Verification items for the finished model (mm, model axes). Round coordinates to 2 decimals unless told otherwise and drop trailing zeros. Write each loop counter-clockwise with the first axis right and the second up, starting at its lowest first coordinate (ties: lowest second). Pieces come first, ordered by that corner, then holes. Notation, with made-up numbers: M 78.25,-4 L 98.25,-4 A15 ccw 98.25,22 Z; hole C 73.5,40 d6. An arc over 180 degrees is marked long. Use a Markdown table: item, result. Add a question column.
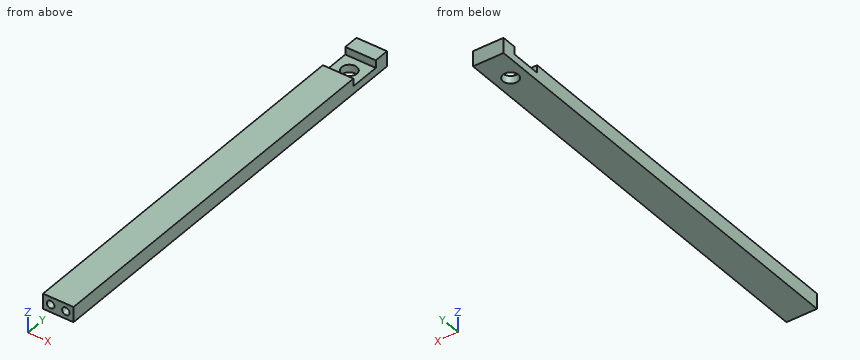
from build123d import *

# Parameters (mm, degrees)
SKETCH1_W           = 25.4
SKETCH1_H           = 12.7
BOSS_EXTRUDE1_DEPTH = 355.6
SKETCH2_W           = 6.35
SKETCH2_H           = 25.4
CUT_EXTRUDE1_DEPTH  = 357.732126392
SKETCH3_R           = 6.35
CUT_EXTRUDE2_DEPTH  = 357.562536591
SKETCH4_R           = 3.175
CUT_EXTRUDE3_DEPTH  = 25.4


with BuildPart() as part:
    # Sketch1 → Boss-Extrude1 (new body)
    with BuildSketch(Plane(origin=(0, 0, 0), x_dir=(1, 0, 0), z_dir=(0, 1, 0))):
        with Locations((12.7, 6.35)):
            Rectangle(SKETCH1_W, SKETCH1_H)
    extrude(amount=BOSS_EXTRUDE1_DEPTH)

    # Sketch2 → Cut-Extrude1 (cut, through all)
    with BuildSketch(Plane(origin=(25.4, 0, 0), x_dir=(0, 0, -1), z_dir=(1, 0, 0))):
        with Locations((3.175, 330.2)):
            Rectangle(SKETCH2_W, SKETCH2_H)
    extrude(amount=-CUT_EXTRUDE1_DEPTH, mode=Mode.SUBTRACT)

    # Sketch3 → Cut-Extrude2 (cut, through all)
    with BuildSketch(Plane.XY.offset(-6.35)):
        with Locations((12.7, 330.2)):
            Circle(SKETCH3_R)
    extrude(amount=-CUT_EXTRUDE2_DEPTH, mode=Mode.SUBTRACT)

    # Sketch4 → Cut-Extrude3 (cut)
    with BuildSketch(Plane.XZ):
        with Locations(Location((6.35, -6.35, 0), (0, 0, 270))):
            Circle(SKETCH4_R)
        with Locations(Location((19.05, -6.35, 0), (0, 0, 270))):
            Circle(SKETCH4_R)
    extrude(amount=-CUT_EXTRUDE3_DEPTH, mode=Mode.SUBTRACT)


solid = part.part
1. Cross-section at A-A on x = 12.7. Enter the section's corners in (y, z).
2. Scan lines: line 1 along X through (y, z) = (18.5, -6.35) (3 decimals); line 2 along X through (y, z) = (330.2, -9); line 3 along Y through (x, z) = (24.75, -3.5). Record each from-to range of solid material in increasing order. Write a range as from..to.
3. Depth check by flat-ended pin: pin 1 Ø5.5 at (x, z) = (19.05, -6.35) entering from -Y. Enter the tip coordinate at first touch or a pass-through.
4. Cross-section at B-B on y = 330.2. Enter the section's corners in (x, z), plus the area to 3 significant figures.
Answer:
| question | item | result |
|---|---|---|
| 1 | outline | M 0,-12.7 L 323.85,-12.7 L 323.85,-6.35 L 317.5,-6.35 L 317.5,0 L 0,0 Z; M 336.55,-12.7 L 355.6,-12.7 L 355.6,0 L 342.9,0 L 342.9,-6.35 L 336.55,-6.35 Z |
| 2 | line 1 | x = 0..3.175, 9.525..15.875, 22.225..25.4 |
| 2 | line 2 | x = 0..6.35, 19.05..25.4 |
| 2 | line 3 | y = 0..317.5, 342.9..355.6 |
| 3 | pin 1 | stops at y = 25.4 |
| 4 | outline | M 0,-12.7 L 6.35,-12.7 L 6.35,-6.35 L 0,-6.35 Z; M 19.05,-12.7 L 25.4,-12.7 L 25.4,-6.35 L 19.05,-6.35 Z |
| 4 | area | 80.6 mm^2 |
